```python
from build123d import *

# Parameters (mm, degrees)
SKETCH1_W          = 50.8
SKETCH1_H          = 31.75
BASE_EXTRUDE_DEPTH = 152.4
CUT_EXTRUDE1_DEPTH = 152.4


with BuildPart() as part:
    # Sketch1 → Base-Extrude (new body)
    with BuildSketch(Plane.XY):
        with Locations((25.4, 15.875)):
            Rectangle(SKETCH1_W, SKETCH1_H)
    extrude(amount=BASE_EXTRUDE_DEPTH)

    # Sketch2 → Cut-Extrude1 (cut)
    with BuildSketch(Plane.XY.offset(152.4)):
        with BuildLine():
            Line((50.8, 6.35), (44.45, 6.35))
            Line((44.45, 6.35), (44.45, 14.605))
            ThreePointArc((44.45, 14.605), (44.821974388, 15.503025612), (45.72, 15.875))
            Line((45.72, 15.875), (49.53, 15.875))
            ThreePointArc((49.53, 15.875), (50.428025612, 16.246974388), (50.8, 17.145))
            Line((50.8, 17.145), (50.8, 20.955))
            ThreePointArc((50.8, 20.955), (50.428025612, 21.853025612), (49.53, 22.225))
            Line((49.53, 22.225), (45.72, 22.225))
            ThreePointArc((45.72, 22.225), (44.821974388, 22.596974388), (44.45, 23.495))
            Line((44.45, 23.495), (44.45, 36.83))
            Line((44.45, 36.83), (54.61, 36.83))
            Line((54.61, 36.83), (54.61, 6.35))
            Line((54.61, 6.35), (50.8, 6.35))
        make_face()
        with BuildLine():
            Line((6.35, 38.1), (6.35, 23.495))
            ThreePointArc((6.35, 23.495), (5.978025612, 22.596974388), (5.08, 22.225))
            Line((5.08, 22.225), (1.27, 22.225))
            ThreePointArc((1.27, 22.225), (0.371974388, 21.853025612), (0, 20.955))
            Line((0, 20.955), (0, 17.145))
            ThreePointArc((0, 17.145), (0.371974388, 16.246974388), (1.27, 15.875))
            Line((1.27, 15.875), (5.08, 15.875))
            ThreePointArc((5.08, 15.875), (5.978025612, 15.503025612), (6.35, 14.605))
            Line((6.35, 14.605), (6.35, 6.35))
            Line((6.35, 6.35), (0, 6.35))
            Line((0, 6.35), (-3.81, 6.35))
            Line((-3.81, 6.35), (-3.81, 38.1))
            Line((-3.81, 38.1), (6.35, 38.1))
        make_face()
    extrude(amount=-CUT_EXTRUDE1_DEPTH, mode=Mode.SUBTRACT)


solid = part.part
```
Check sheet for the modelled part. Datum: model origin and axes. Units: mm. A direction names the side the tool comes from. Round coordinates to 2 decimals unless told otherwise and drop trailing zeros. Write each loop counter-clockwise with the first axis right and the second up, starting at its lowest first coordinate (ties: lowest second). Pieces come first, ordered by that corner, then holes. Notation, with made-up numbers: (52, 45) -> (67, 45) arc R19 ccw to (67, 82) -> close; hole circle Ø6 at (15, 35). An arc over 180 degrees is marked (long way). One line per question, with ' | ' between items. Start each with the question number.
1. Sectioned sample at B-B, the plane y = 11.5. Record the cut outline in (x, z).
2. Set-up check for faces 1 (the face through (44.45, 28, 77)), 2 (the face through (6.35, 11, 77)), 3 (the face through (44.45, 10, 77)): record each of +Z, -Z, +X, -X, +Y, -Y from which the full face is reachable in a straight line by a thin tool's end or side.
3. Scan lines: line 1 along Y through (x, z) = (2.5, 58) (3 decimals); line 2 along X through (y, z) = (14.5, 40); line 3 along X through (y, z) = (21.5, 77). Record each from-to range of solid material in increasing order. Write a range as from..to.
4. Depth check by flat-ended pin: pin 1 (4 mm diameter, centred on y = 11, z = 63.5, fed in from -X); pin 2 (6.5 mm diameter, centred on y = 29.5, z = 84.5, fed in from +X); pin 3 (1.9 mm diameter, centred on x = 3, z = 83, fed in from +Y) (3 decimals). Enter the tip coordinate at first touch or a pass-through.
5. Release check for a two-part mould opening along Y. For faces 4 (the face through (25, 31.75, 75)), 5 (the face through (25, 16, 0)), 6 (the face through (48, 6.35, 77)) record: +Y half, -Y half, draft (parallel to the pull), parting line (faces both ways), or undercut.
6. Sectioned sample at A-A, the plane z = 39. Record the cut outline in (x, y) (3 decimals), then the cut area to 3 significant figures.
Taken from the geometry:
1) outline: (6.35, 0) -> (44.45, 0) -> (44.45, 152.4) -> (6.35, 152.4) -> close
2) face 1: +Z, -Z, +X, +Y | face 2: +Z, -Z, -X | face 3: +Z, -Z, +X
3) line 1: y = 0..6.35, 15.875..22.225 | line 2: x = 6.35..44.45 | line 3: x = 0.12..50.68
4) pin 1: stops at x = 6.35 | pin 2: stops at x = 44.45 | pin 3: stops at y = 22.225
5) face 4: +Y half | face 5: draft | face 6: undercut
6) outline: (0, 0) -> (50.8, 0) -> (50.8, 6.35) -> (44.45, 6.35) -> (44.45, 14.605) arc R1.27 cw to (45.72, 15.875) -> (49.53, 15.875) arc R1.27 ccw to (50.8, 17.145) -> (50.8, 20.955) arc R1.27 ccw to (49.53, 22.225) -> (45.72, 22.225) arc R1.27 cw to (44.45, 23.495) -> (44.45, 31.75) -> (6.35, 31.75) -> (6.35, 23.495) arc R1.27 cw to (5.08, 22.225) -> (1.27, 22.225) arc R1.27 ccw to (0, 20.955) -> (0, 17.145) arc R1.27 ccw to (1.27, 15.875) -> (5.08, 15.875) arc R1.27 cw to (6.35, 14.605) -> (6.35, 6.35) -> (0, 6.35) -> close | area: 1,370 mm^2
